from build123d import *

# Parameters (mm, degrees)
F0_W     = 230
F0_H     = 120.7
F1_DEPTH = 3.7
F2_W     = 230
F2_H     = 1.7
F2_H_2   = 2.5
F3_DEPTH = 2
F4_W     = 230
F4_H     = 10
F5_DEPTH = 0.4
F6_W     = 230
F6_H     = 10
F7_DEPTH = 0.4
F8_W     = 230
F8_H     = 10
F9_DEPTH = 0.4
F11_D    = 3.3
F13_D    = 3.3
F15_D    = 3.3
F17_D    = 1.6
F19_D    = 1.6
F21_D    = 1.6


with BuildPart() as f1:
    # F0 (on Top) → F1 (new body)
    with BuildSketch(Plane.XY):
        Rectangle(F0_W, F0_H)
    extrude(amount=F1_DEPTH)

    # F2 (on face) → F3 (join)
    with BuildSketch(Plane.XY.offset(3.7)):
        with Locations((0, 59.5)):
            Rectangle(F2_W, F2_H)
        with Locations((0, 20.3)):
            Rectangle(F2_W, F2_H_2)
        with Locations((0, -19.4)):
            Rectangle(F2_W, F2_H_2)
        with Locations((0, -59.1)):
            Rectangle(F2_W, F2_H_2)
    extrude(amount=F3_DEPTH)

    # F4 (on face) → F5 (join)
    with BuildSketch(Plane.XY.offset(3.7)):
        with Locations((0, 26.55)):
            Rectangle(F4_W, F4_H)
    extrude(amount=F5_DEPTH)

    # F6 (on face) → F7 (join)
    with BuildSketch(Plane.XY.offset(3.7)):
        with Locations((0, -13.15)):
            Rectangle(F6_W, F6_H)
    extrude(amount=F7_DEPTH)

    # F8 (on face) → F9 (join)
    with BuildSketch(Plane.XY.offset(3.7)):
        with Locations((0, -52.85)):
            Rectangle(F8_W, F8_H)
    extrude(amount=F9_DEPTH)

    # F11 (through all)
    with Locations(Plane.XY.offset(4.1)):
        with Locations((-105, 26.55), (-70, 26.55), (-35, 26.55), (0, 26.55), (35, 26.55), (70, 26.55), (105, 26.55)):
            Hole(F11_D / 2)

    # F13 (through all)
    with Locations(Plane.XY.offset(4.1)):
        with Locations((-105, -13.15), (-70, -13.15), (-35, -13.15), (0, -13.15), (35, -13.15), (70, -13.15), (105, -13.15)):
            Hole(F13_D / 2)

    # F15 (through all)
    with Locations(Plane.XY.offset(4.1)):
        with Locations((-105, -52.85), (-70, -52.85), (-35, -52.85), (0, -52.85), (35, -52.85), (70, -52.85), (105, -52.85)):
            Hole(F15_D / 2)

    # F17 (through all)
    with Locations(Plane.XY.offset(3.7)):
        with Locations((-109, 53.05)):
            Hole(F17_D / 2)

    # F19 (through all)
    with Locations(Plane.XY.offset(3.7)):
        with Locations((-109, 13.35)):
            Hole(F19_D / 2)

    # F21 (through all)
    with Locations(Plane.XY.offset(3.7)):
        with Locations((-109, -26.35)):
            Hole(F21_D / 2)


solid = f1.part
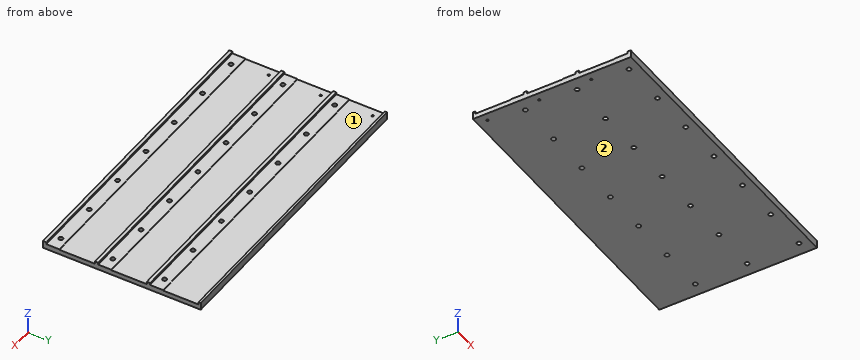
Read the model definition and answer for the solid it produces. Units are mm, in the model's axes. Face numbers are marked on the shaded views. Round coordinates to 2 decimals unless told otherwise and drop trailing zeros. Order: outer loops, then holes, each group sorted by start corner. A loop starts at its lowest first (then second) coordinate and runs counter-clockwise, first axis right, second up.
1) The mould has two halves that part along Y. Classify the marked faces 1 and 2: released by +Y, released by -Y, zero draft, split by the parting line, or undercut.
2) Flat-ended cylindrical pins translate along their axes: pin 1 (3 mm diameter, centred on x = -48, y = 26.5, fed in from +Z); pin 2 (2 mm diameter, centred on x = 70, y = -52.85, fed in from +Z); pin 3 (1.5 mm diameter, centred on x = 49.5, y = -29.5, fed in from +Z). Find the tip coordinate at first contact, or state that the pin passes through.
3) The part is cut by section B-B on y = 45.5. Write down the section's boundary in (x, z), plus the area to 3 significant figures.
4) Straight lines are drawn through the part: L1, parallel to Y at x = 70, z = 2.8; L2, parallel to Y at x = -109, z = 2.45; L3, parallel to Z at x = -56, y = 40. For each, find the intervals that lie inside material, in ascending order.
5) The part is cut by section A-A on x = -54. Write down the section's boundary in (y, z).
Resolved:
1. face 1: undercut
1. face 2: zero draft
2. pin 1: stops at z = 4.1
2. pin 2: passes through
2. pin 3: stops at z = 3.7
3. outline: (-115, 0) - (115, 0) - (115, 3.7) - (-115, 3.7) - close
3. area: 851 mm2
4. L1: y = -60.35 to -54.5, -51.2 to -14.8, -11.5 to 24.9, 28.2 to 60.35
4. L2: y = -60.35 to -27.15, -25.55 to 12.55, 14.15 to 52.25, 53.85 to 60.35
4. L3: z = 0 to 3.7
5. outline: (-60.35, 0) - (60.35, 0) - (60.35, 5.7) - (58.65, 5.7) - (58.65, 3.7) - (31.55, 3.7) - (31.55, 4.1) - (21.55, 4.1) - (21.55, 5.7) - (19.05, 5.7) - (19.05, 3.7) - (-8.15, 3.7) - (-8.15, 4.1) - (-18.15, 4.1) - (-18.15, 5.7) - (-20.65, 5.7) - (-20.65, 3.7) - (-47.85, 3.7) - (-47.85, 4.1) - (-57.85, 4.1) - (-57.85, 5.7) - (-60.35, 5.7) - close
